from build123d import *

# Parameters (mm, degrees)
EXTRUDE_1_DEPTH   = 10
MOVE_BODY_1_ANGLE = 64.736825646
SKETCH_2_R        = 4
EXTRUDE_2_DEPTH   = 3


with BuildPart() as part:
    # 草图1 → 凸台-拉伸1 (new body)
    with BuildSketch(Plane.XY):
        Polygon((7.994684102, 13.847199055), (-7.994684102, 13.847199055), (-15.989368203, 0), (-7.994684102, -13.847199055), (7.994684102, -13.847199055), (15.989368203, 0), align=None)
    extrude(amount=EXTRUDE_1_DEPTH)


with BuildPart() as part_1:
    # Move Body 1: moved
    add(part.part.rotate(Axis((-0.638697904, -1.541953143, 4.361302096), (0.3574067443365927, 0.8628562094610174, 0.3574067443365927)), MOVE_BODY_1_ANGLE))

    # 草图2 → 凸台-拉伸2 (add)
    with BuildSketch(Plane(origin=(-2.133883476, 0.366116524, -1.25), x_dir=(-0.49279927982674293, 0.08455098936288066, 0.8660254037844396), z_dir=(-0.8535533905932747, 0.14644660940672574, -0.49999999999999845))):
        with Locations(Location((4.330127019, 0, 0), (0, 0, 175.096803722))):
            Circle(SKETCH_2_R)
    extrude(amount=EXTRUDE_2_DEPTH)


solid = part_1.part
Work out the finished part from the listing and answer in its coordinate system (mm). Give positions to 0.01 mm unless a question says otherwise; leave off trailing zeros. Loops run counter-clockwise (first coordinate to the right, second up) from the corner with the lowest first, then second, coordinate; pieces in that order, holes last. Notation, with made-up numbers: (6.5, -5.75) - (31.5, -5.75) arc R25 cw to (31.5, 21.25) - close; hole circle Ø3 at (-14.75, -31.75). An arc over 180 degrees is marked (long way). Answer in a Markdown table with one row per item.
(1) Consider L1, parallel to Y at x = 7.75, z = -4; L2, parallel to X at y = 6.5, z = 3.5; L3, parallel to Z at x = -4.5, y = -8. Determine where each line is inside the solid, lowest interval first. Write a range as [from, to].
Results list:
| item | result |
|---|---|
| L1 | y = [-9.62, 9.07] |
| L2 | x = [-3.86, 7.85] |
| L3 | z = [0.34, 18.36] |
(2) Section B-B (x = 0.25) is taken. Give the vertices of the cut face in (y, z) (3 decimals).
Results list:
| item | result |
|---|---|
| outline | (-16.197, 5.03) - (-8.597, -7.945) - (13.241, -1.549) - (16.112, 5.263) - (9.097, 17.238) - (-13.89, 10.505) - close |
(3) For a pull along Y with two mould halves and no side action, classify faces 1 (the face through (-5.084, -11.841, 10.071)), 2 (the face through (-2.032, 11.886, 11.809)), 3 (the face through (-3.08, 5.19, 1.78)) as pulls with the +Y half, pulls with the -Y half, needs draft (parallel to the pull), parting line crosses it, or undercut.
Results list:
| item | result |
|---|---|
| face 1 | pulls with the -Y half |
| face 2 | pulls with the +Y half |
| face 3 | undercut |
(4) Section A-A (z = 14.5) is taken. Give the vertices of the cut face in (x, y), and give its area (3 significant figures).
Results list:
| item | result |
|---|---|
| outline | (-11.19, 1.37) - (-11.08, -7.47) - (-1.66, -11.41) - (2.19, 11.03) - (-9.89, 8.96) - close |
| area | 217 mm² |
(5) Flat-ended cylindrical pins translate along their axes: pin 1 Ø4 at (y, z) = (8.5, 2.5) entering from +X; pin 2 Ø2 at (x, y) = (6.5, 9) entering from +Z; pin 3 Ø8 at (x, z) = (-1.5, 8.5) entering from -Y. Find the tip coordinate at first contact, or state that the pin passes through.
Results list:
| item | result |
|---|---|
| pin 1 | stops at x = 10 |
| pin 2 | stops at z = 8.27 |
| pin 3 | stops at y = -16.38 |
(6) Section C-C (y = 10.5) is taken. Give the vertices of the cut face in (x, z).
Results list:
| item | result |
|---|---|
| outline | (-8.35, 12.32) - (2.36, -5.96) - (9.77, 1.4) - (1.65, 15.25) - close |
(7) Section D-D (x = 5) is taken. Give the vertices of the cut face in (y, z).
Results list:
| item | result |
|---|---|
| outline | (-13.85, 2.41) - (-7.65, -8.18) - (8.51, -8.06) - (15.3, 8.05) - (13.85, 10.52) - close |
